Design review of the part built by this model. Coordinates are the model's own, in mm. A direction names the side the tool comes from. Round coordinates to 2 decimals unless told otherwise and drop trailing zeros. Loops run counter-clockwise (first coordinate to the right, second up) from the corner with the lowest first, then second, coordinate; pieces in that order, holes last. Notation, with made-up numbers: (59.5, 21.5) -> (93.5, 21.5) arc R35 ccw to (93.5, 59.5) -> close; hole circle Ø7 at (-21, 40). An arc over 180 degrees is marked (long way). Answer as CSV lines item,"result". Start each with the question number.
(1) Take a section at B-B, the plane z = 23.5. Write out the cut boundary in (x, y).
(2) Machinability: for faces 5 (the face through (17, 4, 68.43)), 6 (the face through (23.27, 7.52, 100.76)), 7 (the face through (17.642, 2, -85)), which of the approach directions +Z, -Z, +X, -X, +Y, -Y give a long, thin tool a straight path to every point of the face, cutting with its end or side? Answer none if there is none.
(3) Draft analysis for pull direction Y (two halves, no side actions). For faces 1 (the face through (2, 10, 8)), 2 (the face through (-26.358, -26, 5)), 3 (the face through (-10, 7, 101.776)), 4 (the face through (-20.34, -0.7, 7.77)), state which applies: +Y half, -Y half, draft (parallel to the pull), parting line (faces both ways), or undercut.
(4) To check wall thickness, follow line 1 (Z direction, x = -24.75, y = -39.5); line 2 (Z direction, x = -20, y = -39); line 3 (Y direction, x = -2, z = 84). State the ranges of each line that lie inside material, in increasing order. Write a range as from..to.
(5) Take a section at A-A, the plane x = -20.5. State how many separate pieces and enclosed holes the cut face has, and give its area (3 significant figures).
(6) For P1, Ø4, axis at y = -10, z = 76.5, coming from the +X side; P2, Ø12, axis at x = 20.5, z = 10.5, coming from the -Y side; P3, Ø4, axis at x = -20, y = -41.5, coming from the +Z side, all flat-tipped, find the tip position at first contact; note any pin that passes through.
Autodesk Inventor part; units mm, degrees
ref_plane "YZ Plane" through (0, 0, 0) normal (1, 0, 0) x (0, 1, 0)
ref_plane "XZ Plane" through (0, 0, 0) normal (0, 1, 0) x (-1, 0, 0)
ref_plane "XY Plane" through (0, 0, 0) normal (0, 0, 1) x (1, 0, 0)
sketch "Sketch1" plane through (0, 0, 0) normal (0, 1, 0) x (-1, 0, 0)
  line L0 (-32.3469, 68.4305) -> (-32.3469, -55.5695)
  line L1 (-17.6425, -88.9147) -> (-32.3469, -88.9147)
  line L2 (-32.3469, -88.9147) -> (-32.3469, -55.5695)
  line L3 (-32.3469, -55.5695) -> (-17.6425, -55.5695)
  line L4 (-17.6425, -55.5695) -> (-17.6425, -88.9147)
  line L5 (-27.3469, -55.5695) -> (-27.3469, 68.4305)
  line L6 (-32.3469, -55.5695) -> (-27.3469, -55.5695)
  line L7 (-27.3469, -55.5695) -> (-27.3469, 68.4305)
  line L8 (-27.3469, 68.4305) -> (-32.3469, 68.4305)
  line L9 (-32.3469, 68.4305) -> (-32.3469, -55.5695)
  line L10 (-32.3469, 68.4305) -> (-17.6425, 68.4305)
  line L11 (-17.6425, 68.4305) -> (-17.6425, 101.7757)
  line L12 (-17.6425, 101.7757) -> (-32.3469, 101.7757)
  line L13 (-32.3469, 101.7757) -> (-32.3469, 68.4305)
  point P0 (0, 0)
  point P1 (25.2053, -93.5695)
extrude "Extrusion1" add sketch "Sketch1" along normal blind 10
chamfer "Chamfer1" distance 5 angle 45 1 edges at (32.3469, 10, 6.4305)
sketch "Sketch2" plane through (17.6425, 0, -88.9147) normal (-1, 0, 0) x (0, 0, 1)
  line L0 (0, 0) -> (0, 10)
  line L1 (33.3452, 0) -> (33.3452, 10)
  line L2 (0, 10) -> (33.3452, 10)
  line L3 (33.3452, 10) -> (33.3452, 5)
  line L4 (33.3452, 5) -> (0, 5)
  line L5 (0, 5) -> (0, 10)
  line L6 (157.3452, 10) -> (190.6905, 10)
  line L7 (157.3452, 0) -> (157.3452, 10)
  line L8 (190.6905, 10) -> (157.3452, 10)
  line L9 (157.3452, 10) -> (157.3452, 5)
  line L10 (157.3452, 5) -> (190.6905, 5)
  line L11 (190.6905, 5) -> (190.6905, 10)
  point P0 (88.9147, 0)
  dimension "d5" = 5
extrude "Extrusion2" add sketch "Sketch2" along normal blind 46
sketch "Sketch3" plane through (17.6425, 5, -88.9147) normal (0, -1, 0) x (1, 0, 0)
  line L0 (9.7044, 0) -> (-46, 0)
  line L1 (9.7044, 33.3452) -> (-46, 33.3452)
  line L2 (-46, 0) -> (-44, 0)
  line L3 (-44, 0) -> (-44, 33.3452)
  line L4 (-44, 33.3452) -> (-46, 33.3452)
  line L5 (-46, 33.3452) -> (-46, 0)
  line L6 (9.7044, 190.6905) -> (-46, 190.6905)
  line L7 (9.7044, 157.3452) -> (-46, 157.3452)
  line L8 (-46, 190.6905) -> (-45, 190.6905)
  line L9 (-45, 190.6905) -> (-45, 157.3452)
  line L10 (-45, 157.3452) -> (-46, 157.3452)
  line L11 (-46, 157.3452) -> (-46, 190.6905)
  point P0 (-17.6425, 88.9147)
  dimension "d8" = 2
extrude "Extrusion3" add sketch "Sketch3" along normal blind 45
sketch "Sketch4" plane through (27.3469, 0, 68.4305) normal (0, 0, -1) x (-1, 0, 0)
  line L0 (0, 10) -> (55.7044, 10)
  line L1 (0, 0) -> (9.7517, 0)
  line L2 (9.7517, 0) -> (9.7517, 10)
  line L3 (9.7517, 10) -> (0, 10)
  line L4 (0, 10) -> (0, 0)
  line L5 (9.7517, 5) -> (55.7044, 5)
  line L6 (55.7044, 5) -> (55.7044, 10)
  line L7 (55.7044, 10) -> (9.7517, 10)
  line L8 (9.7517, 10) -> (9.7517, 5)
  line L9 (54.7044, 5) -> (54.7044, -40)
  line L10 (55.7044, 5) -> (54.7044, 5)
  line L11 (54.7044, 5) -> (54.7044, -40)
  line L12 (54.7044, -40) -> (55.7044, -40)
  line L13 (55.7044, -40) -> (55.7044, 5)
  point P0 (27.3469, 0)
extrude "Extrusion4" add sketch "Sketch4" along normal blind 150
sketch "Sketch5" plane through (-27.3575, 5, 101.7757) normal (1, 0, 0) x (0, 0, -1)
  line L0 (0, 0) -> (157.3452, 0)
  line L1 (190.6905, -45) -> (157.3452, -45)
  line L2 (0, 0) -> (157.3452, 0)
  line L3 (157.3452, 0) -> (157.3452, -45)
  line L4 (157.3452, -45) -> (0, -45)
  line L5 (0, -45) -> (0, 0)
  point P0 (101.7757, -5)
extrude "Extrusion5" add sketch "Sketch5" along normal blind 1
sketch "Sketch8" plane through (17.6425, -40, -88.9147) normal (0, -1, 0) x (1, 0, 0)
  line L0 (-44, 0) -> (-44, 190.6905)
  line L1 (9.7044, 0) -> (-46, 0)
  line L2 (-44, 190.6905) -> (-46, 190.6905)
  line L3 (-46, 190.6905) -> (-46, 0)
  line L4 (-46, 0) -> (-44, 0)
  line L5 (-44, 0) -> (-44, 190.6905)
  point P0 (-17.6425, 88.9147)
extrude "Extrusion8" add sketch "Sketch8" along normal blind 5
sketch "Sketch9" plane through (-26.3575, 5, 101.7757) normal (1, 0, 0) x (0, 0, -1)
  line L0 (0, 0) -> (0, -50)
  line L1 (0, -50) -> (32, -50)
  line L2 (0, -50) -> (190.6905, -50)
  line L3 (190.6905, -50) -> (158.6905, -50)
  line L4 (32, -50) -> (155.0848, -50)
  line L5 (155.0848, -50) -> (155.0848, -42)
  line L6 (155.0848, -42) -> (32, -42)
  line L7 (32, -42) -> (32, -50)
  point P0 (101.7757, -5)
  dimension "d29" = 32
  dimension "d30" = 32
  dimension "d31" = 8
extrude "Extrusion9" add sketch "Sketch9" along normal blind 10.786
sketch "Sketch10" plane through (-15.5715, 5, 101.7757) normal (1, 0, 0) x (0, 0, -1)
  line L0 (190.6905, 5) -> (0, 5)
  line L1 (95.3452, 5) -> (95.3452, -50)
  line L2 (0, -50) -> (190.6905, -50)
  circle A0 centre (49.4524, -47.1745) radius 1.5
  circle A1 centre (49.4524, -47.1745) radius 1.5
  circle A2 centre (79.4524, -47.1745) radius 1.5
  circle A3 centre (79.4524, -47.1745) radius 1.5
  circle A4 centre (109.4524, -47.1745) radius 1.5
  circle A5 centre (109.4524, -47.1745) radius 1.5
  circle A6 centre (139.4524, -47.1745) radius 1.5
  circle A7 centre (139.4524, -47.1745) radius 1.5
  line L3 (157.7974, -50) -> (157.7974, -40)
  line L4 (31.1074, -40) -> (31.1074, -50)
  line L5 (31.1074, -40) -> (157.7974, -40)
  line L6 (157.7974, -40) -> (157.7974, -50)
  line L7 (157.7974, -50) -> (31.1074, -50)
  line L8 (31.1074, -50) -> (31.1074, -40)
  line L9 (95.3452, -50) -> (95.3452, -40)
  line L10 (155.0848, -42) -> (32, -42)
  line L11 (95.3452, -42) -> (32, -42)
  line L12 (95.3452, -42) -> (158.6902, -42)
  line L13 (158.6902, -42) -> (158.6902, -50)
  line L14 (158.6902, -50) -> (155.0848, -50)
  line L15 (155.0848, -50) -> (155.0848, -42)
  line L16 (155.0848, -50) -> (155.0848, -42)
  line L17 (155.0848, -42) -> (158.6902, -42)
  point P0 (101.7757, -5)
  point P1 (155.0848, -50)
  dimension "d34" = 63.345
extrude "Extrusion10" add sketch "Sketch10" against normal blind 10.786 contours L12 L3 L2 L15 | L12 L13 L2 L3
fillet "Fillet1" radius 5 1 edges at (-28.3575, 10, 6.4305)
fillet "Fillet2" radius 20 1 edges at (-26.3575, 5, 6.4305)
fillet "Fillet4" radius 4 1 edges at (17.5953, 5, -6.5695)
sketch "Sketch11" plane through (0, 10, 0) normal (0, 1, 0) x (1, 0, 0)
  circle A0 centre (23.7073, 85.9487) radius 2
  circle A1 centre (23.7073, 85.9487) radius 1.5
  line L0 (32.3469, -101.7757) -> (32.3469, 88.9147)
  line L1 (32.3469, -6.4305) -> (-25.9991, -6.4305)
  circle A2 centre (23.7073, -98.8097) radius 2
  circle A3 centre (23.7073, -98.8097) radius 1.5
  point P0 (0, 0)
  dimension "d43" = 4
  dimension "d44" = 3
extrude "Extrusion12" cut sketch "Sketch11" against normal blind 4 contours A0 | A1 | A2 | A3
extrude "Extrusion13" cut sketch "Sketch11" against normal blind 100 contours A1 | A3
fillet "Fillet5" radius 1 1 edges at (21.7073, 10, -85.9487)
fillet "Fillet6" radius 1 1 edges at (21.7073, 10, 98.8097)
sketch "Sketch12" plane through (-15.5715, 5, 101.7757) normal (1, 0, 0) x (0, 0, -1)
  line L0 (33.3452, -5) -> (157.3452, -5)
  line L1 (95.3452, -5) -> (95.3452, -50)
  line L2 (94.0723, -38) -> (94.0723, -50)
  line L3 (33.5543, -44.5) -> (157.1905, -44.5)
  circle A0 centre (104.2097, -44.5) radius 1.4
  circle A1 centre (129.8962, -44.5) radius 1.4
  circle A2 centre (86.4808, -44.5) radius 1.4
  circle A3 centre (60.7943, -44.5) radius 1.4
  line L4 (32.0002, -40) -> (158.6902, -40)
  line L5 (158.6902, -50) -> (158.6902, -40)
  line L6 (32.0002, -40) -> (158.6902, -40)
  line L7 (158.6902, -40) -> (158.6902, -50)
  line L8 (158.6902, -50) -> (32.0002, -50)
  line L9 (32.0002, -50) -> (32.0002, -40)
  point P0 (101.7757, -5)
  point P1 (13.9577, -136.3434)
  dimension "d52" = 2.8
  dimension "d53" = 2.8
extrude "Extrusion14" cut sketch "Sketch12" against normal blind 100 contours A1 L3 | L3 A1 | A0 L3 | L3 A0 | A3 L3 | L3 A3 | A2 L3 | L3 A2
properties part number "bumper belakang"
The answers:
1,outline,"(-28.36, -45) -> (-15.57, -45) -> (-15.57, -37) -> (-26.36, -37) -> (-26.36, -15) arc R20 cw to (-6.36, 5) -> (13.6, 5) arc R4 cw to (17.6, 1) -> (17.6, 0) -> (32.35, 0) -> (32.35, 5) -> (27.35, 10) -> (-23.36, 10) arc R5 ccw to (-28.36, 5) -> close"
2,face 5,"+Z, -Y"
2,face 6,"+Y"
2,face 7,"-Z, -Y"
3,face 1,"+Y half"
3,face 2,"undercut"
3,face 3,"draft"
3,face 4,"undercut"
4,line 1,"-56.91..-29.52, -26.72..-3.83, -1.03..13.89, 16.69..39.58, 42.38..69.78"
4,line 2,"-56.91..-29.43, -26.81..-3.74, -1.13..13.99, 16.6..39.67, 42.29..69.78"
4,line 3,"5..10"
5,separate pieces,"2"
5,enclosed holes,"4"
5,area,"3,060 mm²"
6,P1,"x = -25.09"
6,P2,"y = 0"
6,P3,"z = 69.78"
